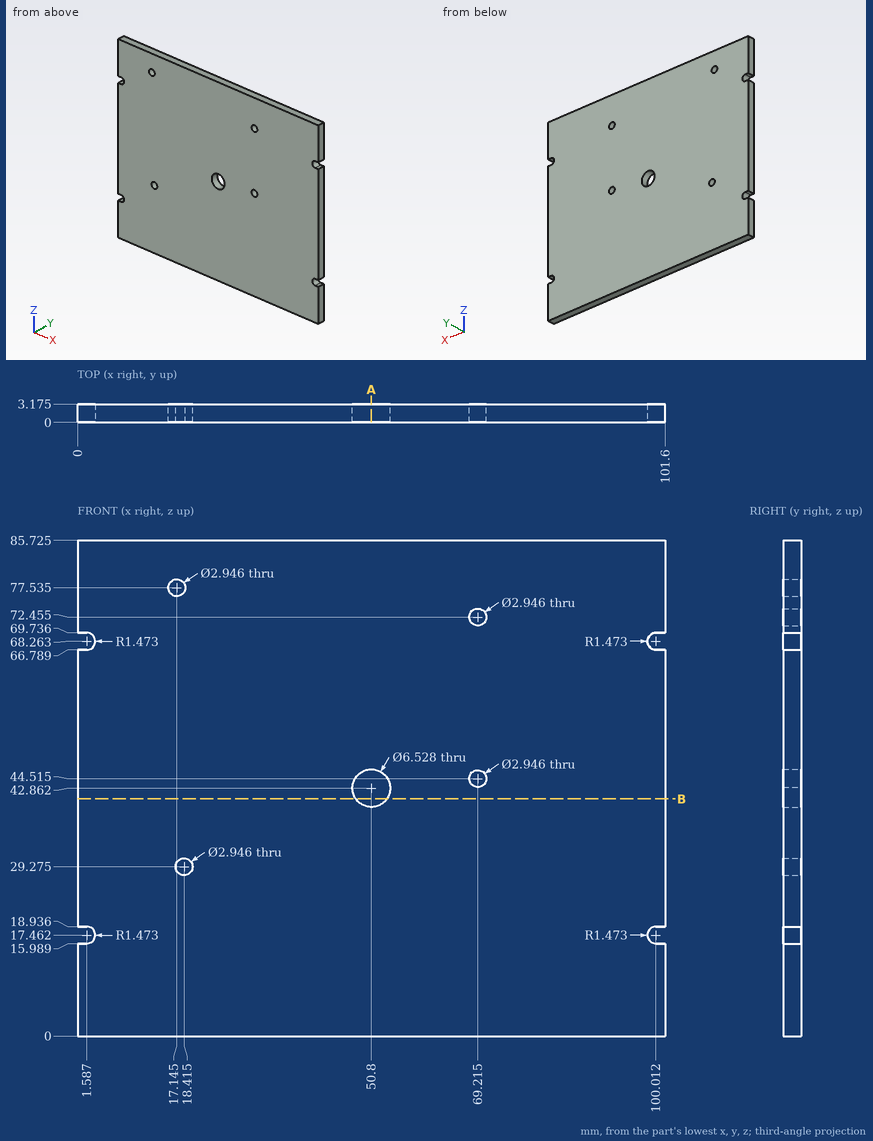
Study the drawing (mm; zero at the part's minimum x, y, z) and answer. Round coordinates to 2 decimals unless told otherwise and drop trailing zeros. Write each loop counter-clockwise with the first axis right and the second up, starting at its lowest first coordinate (ties: lowest second). Pieces come first, ordered by that corner, then holes. Notation, with made-up numbers: (84, -37) - (140, -37) arc R28 ccw to (140, -18) - close; hole circle Ø6 at (79, 81). An arc over 180 degrees is marked (long way). Return JSON: item names as keys, results as strings. Group by question number.
Q1. The part is cut by section A-A on x = 50.8. Write down the section's boundary in (y, z) (1 decimal).
Q2. The part is cut by section B-B on z = 41. Write down the section's boundary in (x, y) (1 decimal).
Q3. This flat-tipped pin is pushed along its axis until it touches: pin 1 Ø1.7 at (x, y) = (1, 2) entering from -Z. Where does it stop, or does it pass through?
Q4. Find the intervals of material crossed by L1, parallel to Z at x = 68.5, y = 1.95 (1 decimal); L2, parallel to X at y = 0.8, z = 29; L3, parallel to X at y = 2.85, z = 40 (1 decimal), in increasing order.
Solved:
{
 "1": {"outline": "(0, 0) - (3.2, 0) - (3.2, 39.6) - (0, 39.6) - close; (0, 46.1) - (3.2, 46.1) - (3.2, 85.7) - (0, 85.7) - close"},
 "2": {"outline": "(0, 0) - (48.1, 0) - (48.1, 3.2) - (0, 3.2) - close; (53.5, 0) - (101.6, 0) - (101.6, 3.2) - (53.5, 3.2) - close"},
 "3": {"pin 1": "z = 0"},
 "4": {"L1": "0 to 43.2, 45.8 to 71.2, 73.7 to 85.7", "L2": "0 to 16.97, 19.86 to 101.6", "L3": "0 to 49.2, 52.4 to 101.6"}
}
